```python
from build123d import *

# Parameters (mm, degrees)
SKETCH1_W                  = 10
SKETCH1_H                  = 10
BOSS_EXTRUDE1_DEPTH        = 15
SKETCH2_R                  = 1
CUT_EXTRUDE1_DEPTH         = 6
SKETCH3_R                  = 1
CUT_EXTRUDE2_DEPTH         = 6
CHAMFER1_SIZE              = 0.2
LPATTERN2_COUNT            = 3
LPATTERN2_PITCH            = 10
CHAMFER1_OF_LPATTERN2_SIZE = 0.2
SKETCH4_R                  = 0.95
CUT_EXTRUDE3_DEPTH         = 7
CHAMFER2_SIZE              = 0.2
CHAMFER3_SIZE              = 0.1


with BuildPart() as part:
    # Sketch1 → Boss-Extrude1 (new body, symmetric)
    with BuildSketch(Plane(origin=(0, 0, 0), x_dir=(0, 0, -1), z_dir=(1, 0, 0))):
        Rectangle(SKETCH1_W, SKETCH1_H)
    extrude(amount=BOSS_EXTRUDE1_DEPTH, both=True)

    # Sketch2 → Cut-Extrude1 (cut, symmetric)
    with BuildSketch(Plane.XY):
        with Locations((-12.5, 0)):
            Circle(SKETCH2_R)
        with Locations((-7.5, 0)):
            Circle(SKETCH2_R)
    cut_extrude1 = extrude(amount=CUT_EXTRUDE1_DEPTH, both=True, mode=Mode.SUBTRACT)

    # Sketch3 → Cut-Extrude2 (cut, symmetric)
    with BuildSketch(Plane(origin=(0, 0, 0), x_dir=(1, 0, 0), z_dir=(0, 1, 0))):
        with Locations(Location((-10, 2.5, 0), (0, 0, 270))):  # turned: the seam where the file's is
            Circle(SKETCH3_R)
        with Locations(Location((-10, -2.5, 0), (0, 0, 270))):  # turned: the seam where the file's is
            Circle(SKETCH3_R)
    cut_extrude2 = extrude(amount=CUT_EXTRUDE2_DEPTH, both=True, mode=Mode.SUBTRACT)

    # Chamfer1
    chamfer1_edges = [part.edges().sort_by_distance(p)[0] for p in [
        (-13.5, 0, -5),
        (-13.5, 0, 5),
        (-8.5, 0, -5),
        (-8.5, 0, 5),
        (-10, -5, -3.5),
        (-10, 5, -3.5),
        (-10, -5, 1.5),
        (-10, 5, 1.5),
    ]]
    chamfer(chamfer1_edges, length=CHAMFER1_SIZE)

    # LPattern2: Cut-Extrude1, Cut-Extrude2 ×3
    with Locations(*[(i * LPATTERN2_PITCH, 0, 0) for i in range(1, LPATTERN2_COUNT)]):
        add(cut_extrude1, mode=Mode.SUBTRACT)
        add(cut_extrude2, mode=Mode.SUBTRACT)

    # Chamfer1 of LPattern2
    chamfer1_of_lpattern2_edges = [part.edges().sort_by_distance(p)[0] for p in [
        (-3.5, 0, -5),
        (-3.5, 0, 5),
        (1.5, 0, -5),
        (1.5, 0, 5),
        (0, -5, -3.5),
        (0, 5, -3.5),
        (0, -5, 1.5),
        (0, 5, 1.5),
        (6.5, 0, -5),
        (6.5, 0, 5),
        (11.5, 0, -5),
        (11.5, 0, 5),
        (10, -5, -3.5),
        (10, 5, -3.5),
        (10, -5, 1.5),
        (10, 5, 1.5),
    ]]
    chamfer(chamfer1_of_lpattern2_edges, length=CHAMFER1_OF_LPATTERN2_SIZE)

    # Sketch4 → Cut-Extrude3 (cut)
    with BuildSketch(Plane.ZY.offset(15)):
        with Locations((0, 2.5)):
            Circle(SKETCH4_R)
        with Locations((0, -2.5)):
            Circle(SKETCH4_R)
    cut_extrude3 = extrude(amount=-CUT_EXTRUDE3_DEPTH, mode=Mode.SUBTRACT)

    # Mirror1: Cut-Extrude3 across plane
    add(cut_extrude3.mirror(Plane(origin=(0, 0, 0), x_dir=(0, 0, 1), z_dir=(1, 0, 0))), mode=Mode.SUBTRACT)

    # Chamfer2
    chamfer2_edges = [part.edges().sort_by_distance(p)[0] for p in [
        (15, 0, -5),
        (15, 5, 0),
        (15, 0, 5),
        (-15, 5, 0),
        (-15, 0, -5),
        (-15, -5, 0),
        (-15, 0, 5),
        (15, -5, 0),
        (0, 5, 5),
        (0, 5, -5),
        (0, -5, -5),
        (0, -5, 5),
    ]]
    chamfer(chamfer2_edges, length=CHAMFER2_SIZE)

    # Chamfer3
    chamfer3_edges = [part.edges().sort_by_distance(p)[0] for p in [
        (-15, 2.5, -0.95),
        (-15, -2.5, -0.95),
        (15, 2.5, -0.95),
        (15, -2.5, -0.95),
    ]]
    chamfer(chamfer3_edges, length=CHAMFER3_SIZE)


solid = part.part
```
Could you check a few things on this model? Use its own coordinates, in mm. A direction names the side the tool comes from. Round coordinates to 2 decimals unless told otherwise and drop trailing zeros. Write each loop counter-clockwise with the first axis right and the second up, starting at its lowest first coordinate (ties: lowest second). Pieces come first, ordered by that corner, then holes. Notation, with made-up numbers: M 68,65 L 122,65 A10 cw 122,74 Z; hole C -7,25 d8. An arc over 180 degrees is marked long. Answer in a Markdown table with one row per item. Add a question column.
Q1. On a 3-axis mill with a long thin cutter (end or side, diameter ignored), from which of +Z, -Z, +X, -X, +Y, -Y can I reach the whole of each face in a straight line? I mean faces 3 (the flat face through (0, 0, -5)), 4 (the cylindrical face through (-11.498, 3.442, -0.124)). Say none if no direction works.
Q2. Imagine slicing it at B-B (z = -4). Please give me the cut outline in (x, y), then the cut area to 3 significant figures.
Q3. If I drill on line 1 (X direction, y = -3.75, z = 2.5); line 2 (Z direction, x = -10.5, y = -4.25); line 3 (Y direction, x = 2.5, z = 0.5), over which ranges is the centre line in solid material (lowest first)? Write a range as from..to.
Q4. Imagine slicing it at C-C (x = 2.5). Please give me the cut outline in (y, z).
Q5. Will these pins go through, and if not, where does the flat tip stop? pin 1 Ø2 at (y, z) = (-2.5, 0) entering from -X; pin 2 Ø1.7 at (y, z) = (2.5, 0) entering from -X.
Q6. If we mould it in two halves opening along Y, with no side actions, what happens to faces 1 (the flat face through (-15, 0, 0)), 2 (the flat face through (8, -2, 0))? For each: +Y half, -Y half, draft (parallel to the pull), parting line (faces both ways), or undercut.
Q7. Imagine slicing it at D-D (y = 2.5). Please give me the cut outline in (x, z).
Q8. Imagine slicing it at A-A (x = 12.5). Please give me the cut outline in (y, z), then the cut area to 3 significant figures.
Values:
| question | item | result |
|---|---|---|
| 1 | face 3 | -Z, +X, -X, +Y, -Y |
| 1 | face 4 | -X |
| 2 | outline | M -15,-4.8 L -14.8,-5 L 14.8,-5 L 15,-4.8 L 15,4.8 L 14.8,5 L -14.8,5 L -15,4.8 Z; hole C -12.5,0 d2; hole C -7.5,0 d2; hole C -2.5,0 d2; hole C 2.5,0 d2; hole C 7.5,0 d2; hole C 12.5,0 d2 |
| 2 | area | 281 mm^2 |
| 3 | line 1 | -15..-11, -9..-1, 1..9, 11..15 |
| 3 | line 2 | -5..-3.37, -1.63..1.63, 3.37..5 |
| 3 | line 3 | -5..-1, 1..5 |
| 4 | outline | M -5,-4.8 L -4.8,-5 L -1.2,-5 L -1,-4.8 L -1,4.8 L -1.2,5 L -4.8,5 L -5,4.8 Z; M 1,-4.8 L 1.2,-5 L 4.8,-5 L 5,-4.8 L 5,4.8 L 4.8,5 L 1.2,5 L 1,4.8 Z |
| 5 | pin 1 | x = -14.95 |
| 5 | pin 2 | x = -8 |
| 6 | face 1 | draft |
| 6 | face 2 | undercut |
| 7 | outline | M -15,-4.8 L -14.8,-5 L 14.8,-5 L 15,-4.8 L 15,-1.05 L 14.9,-0.95 L 8,-0.95 L 8,0.95 L 14.9,0.95 L 15,1.05 L 15,4.8 L 14.8,5 L -14.8,5 L -15,4.8 L -15,1.05 L -14.9,0.95 L -8,0.95 L -8,-0.95 L -14.9,-0.95 L -15,-1.05 Z; hole C -10,-2.5 d2; hole C -10,2.5 d2; hole C 0,-2.5 d2; hole C 0,2.5 d2; hole C 10,-2.5 d2; hole C 10,2.5 d2 |
| 8 | outline | M -5,-4.8 L -4.8,-5 L -1.2,-5 L -1,-4.8 L -1,4.8 L -1.2,5 L -4.8,5 L -5,4.8 Z; M 1,-4.8 L 1.2,-5 L 4.8,-5 L 5,-4.8 L 5,4.8 L 4.8,5 L 1.2,5 L 1,4.8 Z; hole C -2.5,0 d1.9; hole C 2.5,0 d1.9 |
| 8 | area | 74.2 mm^2 |
